Design review of the part built by this model. Coordinates are the model's own, in mm. A direction names the side the tool comes from. Coordinates: 2 decimals unless noted, no trailing zeros. Write each loop counter-clockwise with the first axis right and the second up, starting at its lowest first coordinate (ties: lowest second). Pieces come first, ordered by that corner, then holes.
```python
from build123d import *

# Parameters (mm, degrees)
F0_R     = 73.025
F1_DEPTH = 69.85
F3_DEPTH = 68.834
F4_R     = 5.08


with BuildPart() as f1:
    # F0 (on Top) → F1 (new body)
    with BuildSketch(Plane.XY):
        Circle(F0_R)
    extrude(amount=F1_DEPTH)

    # F2 (on face) → F3 (cut)
    with BuildSketch(Plane.XY.offset(69.85)):
        with BuildLine():
            Line((-9.652, 0), (-9.652, 59.5478338901))
            ThreePointArc((-9.652, 59.5478338901), (-60.325, 0), (-9.652, -59.5478338901))
            Line((-9.652, -59.5478338901), (-9.652, 0))
        make_face()
        with BuildLine():
            ThreePointArc((9.652, -59.5478338901), (45.9421512611, -39.0950682631), (60.325, 0))
            ThreePointArc((60.325, 0), (45.9421512611, 39.0950682631), (9.652, 59.5478338901))
            Line((9.652, 59.5478338901), (9.652, 0))
            Line((9.652, 0), (9.652, -59.5478338901))
        make_face()
    extrude(amount=-F3_DEPTH, mode=Mode.SUBTRACT)

    # F4
    f4_edges = [f1.edges().sort_by_distance(p)[0] for p in [
        (-73.025, 0, 69.85),
        (9.652, 0, 69.85),
        (60.325, 0, 69.85),
        (-9.652, 0, 69.85),
        (-60.325, 0, 69.85),
        (-73.025, 0, 0),
    ]]
    fillet(f4_edges, radius=F4_R)


solid = f1.part
```
(1) For faces 4 (the flat face through (0, 0, 69.85)), 5 (the flat face through (9.652, 1, 33)), list the 3-axis set-ups (+Z, -Z, +X, -X, +Y, -Y) from which the entire face can be reached by the end or side of a thin tool; tool diameter is ignored.
(2) Insertion check: pin 1 Ø1 at (x, y) = (-26.5, 3.5) entering from +Z; pin 2 Ø8 at (x, z) = (-29, 12.5) entering from +Y; pin 3 Ø1 at (x, z) = (-46, 39) entering from -Y. Each pin has a flat end and moves straight along its axis. Give the tip position at first contact, or say it passes through.
(3) Mouldability with a two-part tool opening along X and no side actions: class faces 1 (the cylindrical face through (69.653, 21.935, 34.507)), 2 (the flat face through (-1, 1, 0)), 3 (the cylindrical face through (-60.313, 1.191, 33.339)) as +X half, -X half, draft (parallel to the pull), parting line (faces both ways), or undercut.
(4) Wall thickness on line 1 (X direction, y = -1.5, z = 20); line 2 (X direction, y = -48.5, z = 51); line 3 (Z direction, x = 24, y = -53): over which ranges is each line inside the solid? List them lowest first.
(5) Consider section A-A (z = 12). Give the boundary of the cut face in (x, y) (3 decimals).
Results:
1. face 4: +Z, +X, -X, +Y, -Y
1. face 5: +Z
2. pin 1: stops at z = 1.02
2. pin 2: stops at y = 68.61
2. pin 3: stops at y = -57.12
3. face 1: parting line
3. face 2: draft
3. face 3: undercut
4. line 1: x = -73.01 to -60.31, -9.65 to 9.65, 60.31 to 73.01
4. line 2: x = -54.59 to -35.87, -9.65 to 9.65, 35.87 to 54.59
4. line 3: z = 0 to 1.02
5. outline: circle Ø146.05 at (0, 0); hole (-9.652, -59.548) - (-9.652, 59.548) arc R60.325 ccw to start; hole (9.652, -59.548) arc R60.325 ccw to (9.652, 59.548) - close
